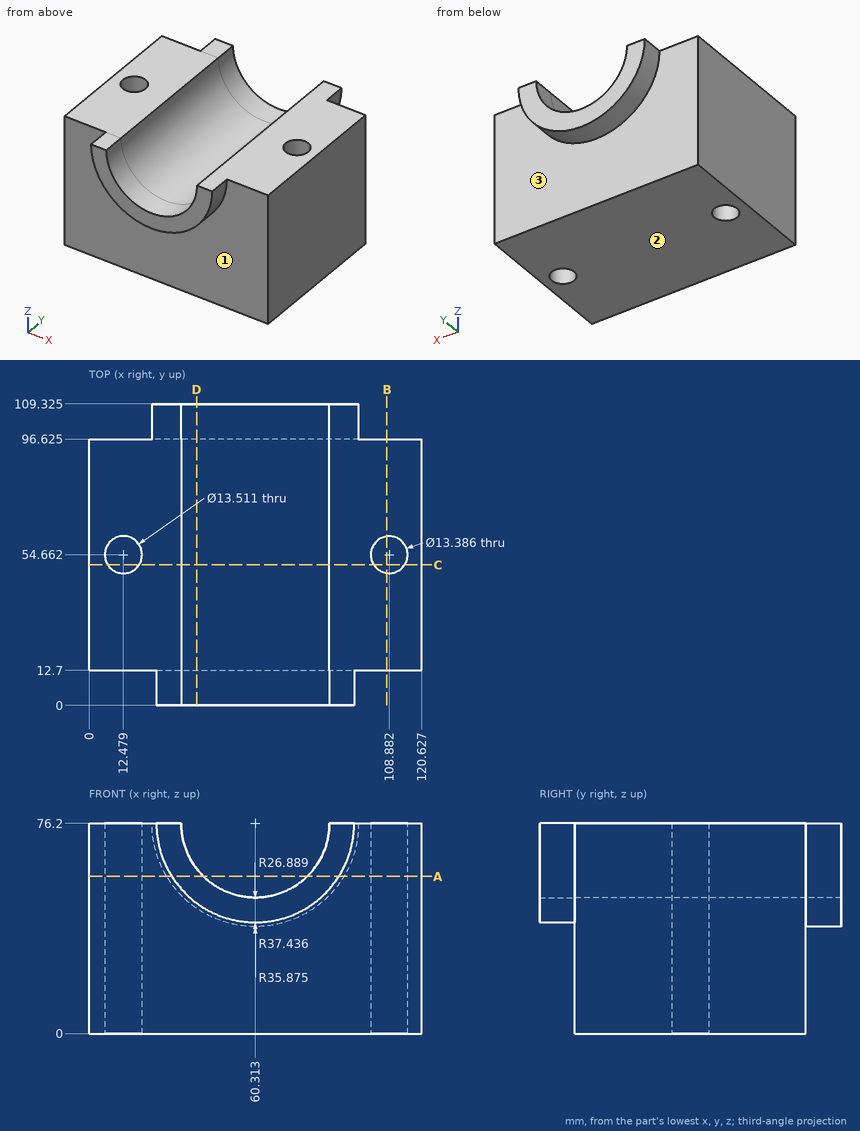
Here's the drawing with two shaded views (mm, measured from the low corner). I have some questions. A direction names the side the tool comes from. Round coordinates to 2 decimals unless told otherwise and drop trailing zeros. Order: outer loops, then holes, each group sorted by start corner. A loop starts at its lowest first (then second) coordinate and runs counter-clockwise, first axis right, second up. Notation, with made-up numbers: (65, 24.25) -> (91, 24.25) arc R26 ccw to (91, 50.25) -> close; hole circle Ø6 at (7.5, 28.25). An arc over 180 degrees is marked (long way). Write each question's results on one line, items separated by ' | '. Start each with the question number.
Item 1: If we section it at D-D, the plane x = 39: Write out the boundary of the cut face in (y, z) (1 decimal).
Item 2: If we section it at A-A, the plane z = 57: Write out the boundary of the cut face in (x, y) (1 decimal).
Item 3: If we section it at C-C, the plane y = 51: Write out the boundary of the cut face in (x, z) (1 decimal).
Item 4: Will these pins go through, and if not, where does the flat tip stop? pin 1 (1 mm diameter, centred on x = 77.5, z = 17.5, fed in from +Y) (1 decimal); pin 2 (10.5 mm diameter, centred on x = 108.88, y = 54.66, fed in from -Z); pin 3 (10 mm diameter, centred on x = 54, y = 97.5, fed in from +Z); pin 4 (21.5 mm diameter, centred on x = 12.48, y = 54.66, fed in from +Z).
Item 5: Please list where these lines run through material, in increasing order: L1, parallel to X at y = 52, z = 9.5; L2, parallel to Y at x = 56.5, z = 7.5 (1 decimal); L3, parallel to X at y = 17.5, z = 69.5 (1 decimal).
Item 6: Which directions (+Z, -Z, +X, -X, +Y, -Y) give clear straight access to the entire face, cutting with the end or side of a thin tool? Please do the marked faces 1, 2 and 3.
Item 7: If we section it at B-B, the plane x = 108: Write out the boundary of the cut face in (y, z) (1 decimal), then the cut area to 3 significant figures.
Results:
1) outline: (0, 47.3) -> (12.7, 47.3) -> (12.7, 0) -> (96.6, 0) -> (96.6, 45.4) -> (109.3, 45.4) -> (109.3, 59.8) -> (0, 59.8) -> close
2) outline: (0, 12.7) -> (30, 12.7) -> (30, 0) -> (41.5, 0) -> (41.5, 109.3) -> (28.2, 109.3) -> (28.2, 96.6) -> (0, 96.6) -> close; (79.1, 0) -> (90.6, 0) -> (90.6, 12.7) -> (120.6, 12.7) -> (120.6, 96.6) -> (92.5, 96.6) -> (92.5, 109.3) -> (79.1, 109.3) -> close; hole circle Ø13.5 at (12.5, 54.7); hole circle Ø13.4 at (108.9, 54.7)
3) outline: (0, 0) -> (6.8, 0) -> (6.8, 76.2) -> (0, 76.2) -> close; (18.2, 0) -> (103.3, 0) -> (103.3, 76.2) -> (87.2, 76.2) arc R26.9 cw to (33.4, 76.2) -> (18.2, 76.2) -> close; (114.5, 0) -> (120.6, 0) -> (120.6, 76.2) -> (114.5, 76.2) -> close
4) pin 1: stops at y = 96.6 | pin 2: passes through | pin 3: stops at z = 51.81 | pin 4: stops at z = 76.2
5) L1: x = 0 to 6.27, 18.69 to 102.74, 115.02 to 120.63 | L2: y = 12.7 to 96.6 | L3: x = 0 to 34.3, 86.4 to 120.6
6) face 1: -Z, -Y | face 2: -Z, +X, -X, +Y, -Y | face 3: -Z, +Y
7) outline: (12.7, 0) -> (48, 0) -> (48, 76.2) -> (12.7, 76.2) -> close; (61.3, 0) -> (96.6, 0) -> (96.6, 76.2) -> (61.3, 76.2) -> close | area: 5,380 mm2
